Source: CAD feature listing. Evaluate the final solid. Frame: model axes, mm. A direction names the side the tool comes from. Give positions to 0.01 mm unless a question says otherwise; leave off trailing zeros. Write each loop counter-clockwise with the first axis right and the second up, starting at its lowest first coordinate (ties: lowest second). Pieces come first, ordered by that corner, then holes. Notation, with made-up numbers: (-28.5, 70) -> (27.5, 70) arc R12 cw to (27.5, 90) -> close; hole circle Ø1 at (47, 71). An arc over 180 degrees is marked (long way). Use a Markdown table: item, result. Add a question column.
Autodesk Inventor part; units mm, degrees
ref_plane "YZ Plane" through (0, 0, 0) normal (1, 0, 0) x (0, 1, 0)
ref_plane "XZ Plane" through (0, 0, 0) normal (0, 1, 0) x (-1, 0, 0)
ref_plane "XY Plane" through (0, 0, 0) normal (0, 0, 1) x (1, 0, 0)
sketch "Sketch1" plane through (0, 0, 0) normal (0, 0, 1) x (1, 0, 0)
  line L0 (0, 0) -> (20, 0)
  line L1 (20, 0) -> (20, 10)
  line L2 (20, 10) -> (0, 10)
  line L3 (0, 10) -> (0, 0)
  line L4 (5.5, 0) -> (14.5, 0)
  line L5 (14.5, 0) -> (14.5, 4)
  line L6 (14.5, 4) -> (5.5, 4)
  line L7 (5.5, 4) -> (5.5, 0)
  point P0 (10, 4)
  point P1 (10, 10)
  dimension "d0" = 9
  dimension "d1" = 4
  dimension "d2" = 10
  dimension "d3" = 20
extrude "Extrusion1" add sketch "Sketch1" along normal blind 40.5 contours L3 L2 L1 L0 L5 L6 L7
properties part number "MGN9H"
(1) Access query for faces 5 (the flat face through (14.5, 2, 20)), 6 (the flat face through (10, 10, 20)). Directions: +Z, -Z, +X, -X, +Y, -Y. A direction counts if a zero-diameter tool reaches every point of the face in a straight line with its end or side. Return the directions, or none.
(2) Cut plane B-B on z = 37.5. Return the cut outline in (x, y).
(3) First-contact query: pin 1 Ø4.5 at (x, z) = (8, 20) entering from -Y. Flat tip, straight axial feed; report the tip coordinate or a pass-through.
(4) Material intervals for L1, parallel to X at y = 3, z = 13; L2, parallel to Y at x = 13.5, z = 17.5, sorted ascending.
(5) Cut plane C-C on x = 10.25. Return the cut outline in (y, z).
(6) Mould query, pull axis X, two halves, no side actions, for faces 1 (the flat face through (0, 5, 20)), 2 (the flat face through (10, 6, 0)), 3 (the flat face through (20, 5, 20)), 4 (the flat face through (5.5, 2, 20)). Classes: +X half, -X half, draft (parallel to the pull), parting line (faces both ways), or undercut.
(7) Cut plane A-A on y = 2.5. Return the cut outline in (x, z), then the cut area to 4 significant figures.
Output:
| question | item | result |
|---|---|---|
| 1 | face 5 | +Z, -Z, -Y |
| 1 | face 6 | +Z, -Z, +X, -X, +Y |
| 2 | outline | (0, 0) -> (5.5, 0) -> (5.5, 4) -> (14.5, 4) -> (14.5, 0) -> (20, 0) -> (20, 10) -> (0, 10) -> close |
| 3 | pin 1 | y = 4 |
| 4 | L1 | 0 to 5.5, 14.5 to 20 |
| 4 | L2 | 4 to 10 |
| 5 | outline | (4, 0) -> (10, 0) -> (10, 40.5) -> (4, 40.5) -> close |
| 6 | face 1 | -X half |
| 6 | face 2 | draft |
| 6 | face 3 | +X half |
| 6 | face 4 | undercut |
| 7 | outline | (0, 0) -> (5.5, 0) -> (5.5, 40.5) -> (0, 40.5) -> close; (14.5, 0) -> (20, 0) -> (20, 40.5) -> (14.5, 40.5) -> close |
| 7 | area | 445.5 mm^2 |
